Autodesk Inventor part; units mm, degrees
ref_plane "YZ Plane" through (0, 0, 0) normal (1, 0, 0) x (0, 1, 0)
ref_plane "XZ Plane" through (0, 0, 0) normal (0, 1, 0) x (-1, 0, 0)
ref_plane "XY Plane" through (0, 0, 0) normal (0, 0, 1) x (1, 0, 0)
sketch "Эскиз1" plane through (0, 0, 0) normal (0, 1, 0) x (-1, 0, 0)
  line L0 (30, 60) -> (-30, 60)
  line L1 (-30, 60) -> (-30, -60)
  line L2 (-30, -60) -> (30, -60)
  line L3 (30, -60) -> (30, 60)
  point P0 (0, 0)
  dimension "d0" = 60
  dimension "d1" = 120
extrude "Выдавливание1" add sketch "Эскиз1" along normal blind 80
sketch "Эскиз2" plane through (0, 0, 0) normal (1, 0, 0) x (0, 1, 0)
  line L0 (80, 60) -> (80, -60)
  line L1 (80, -30) -> (70, -30)
  line L2 (80, -30) -> (90, -30) construction
  line L3 (70, -30) -> (70, -10)
  line L4 (70, -10) -> (60, -10)
  line L5 (60, -10) -> (60, 10)
  line L6 (60, 10) -> (70, 10)
  line L7 (70, 10) -> (70, 30)
  line L8 (70, 30) -> (80, 30)
extrude "Выдавливание2" cut sketch "Эскиз2" against normal mid plane 80
sketch "Эскиз3" plane through (0, 0, 0) normal (1, 0, 0) x (0, 1, 0)
  line L0 (0, 60) -> (0, -60)
  line L1 (0, -15) -> (10, -15)
  line L2 (0, -15) -> (10, -15) construction
  line L3 (10, -15) -> (10, -25)
  line L4 (10, -25) -> (15, -25)
  line L5 (0, -15) -> (0, 15)
  line L6 (0, 15) -> (10, 15)
  line L7 (10, 15) -> (10, 25)
  line L8 (10, 25) -> (15, 25)
  arc A0 (15, -25) -> (15, 25) centre (15, 0) ccw
  point P0 (0, 0)
  dimension "d20" = 10
  dimension "d21" = 0
  dimension "d22" = 30
extrude "Выдавливание3" cut sketch "Эскиз3" against normal mid plane 80
sketch "Эскиз4" plane through (0, 0, 0) normal (0, 1, 0) x (-1, 0, 0)
  circle A0 centre (0, 0) radius 25
  dimension "d25" = 50
extrude "Выдавливание4" cut sketch "Эскиз4" along normal blind 80
sketch "Эскиз5" plane through (30, 0, -60) normal (1, 0, 0) x (0, 0, -1)
  line L0 (-120, 0) -> (-120, 80)
  line L1 (-120, 20) -> (-100, 20)
  line L2 (-120, 20) -> (-100, 20) construction
  line L3 (-100, 20) -> (-100, 80)
  line L4 (-120, 80) -> (-90, 80)
  line L5 (0, 0) -> (0, 80)
  line L6 (0, 20) -> (-20, 20)
  line L7 (0, 20) -> (20, 20) construction
  line L8 (-20, 20) -> (-20, 80)
  line L9 (0, 80) -> (-30, 80)
  point P0 (-60, 0)
  dimension "d28" = 20
  dimension "d29" = 0
  dimension "d30" = 20
  dimension "d31" = 180
extrude "Выдавливание5" cut sketch "Эскиз5" against normal blind 25
sketch "Эскиз6" plane through (-30, 0, 60) normal (-1, 0, 0) x (0, 0, 1)
  line L0 (-120, 0) -> (-120, 80)
  line L1 (-120, 20) -> (-100, 20)
  line L2 (-120, 20) -> (-100, 20)
  line L3 (-100, 20) -> (-100, 80)
  line L4 (-120, 80) -> (-90, 80)
  line L5 (-20, 20) -> (0, 20)
  line L6 (0, 20) -> (-20, 20)
  line L7 (-20, 80) -> (-20, 20)
  line L8 (-20, 20) -> (-20, 80)
  line L9 (-20, 80) -> (-30, 80)
  line L10 (-30, 80) -> (0, 80)
  line L11 (-20, 80) -> (0, 80)
  line L12 (0, 20) -> (0, 80)
  line L13 (0, 80) -> (0, 20)
  point P0 (-60, 0)
extrude "Выдавливание6" cut sketch "Эскиз6" against normal blind 25
sketch "Эскиз7" plane through (5, 0, -60) normal (1, 0, 0) x (0, 0, -1)
  line L0 (-20, 80) -> (-20, 20)
  line L1 (-20, 20) -> (0, 20)
  line L2 (-20, 80) -> (0, 20)
  line L3 (0, 20) -> (-20, 20)
  line L4 (0, 80) -> (-20, 80)
  line L5 (-20, 20) -> (-20, 80)
  line L6 (0, 20) -> (0, 80)
  line L7 (0, 80) -> (0, 20)
  point P0 (-60, 0)
extrude "Выдавливание7" cut sketch "Эскиз7" against normal blind 25 contours L4 L6 L2
sketch "Эскиз8" plane through (5, 0, -60) normal (1, 0, 0) x (0, 0, -1)
  line L0 (-120, 20) -> (-120, 80)
  line L1 (-100, 80) -> (-120, 20)
  line L2 (-120, 20) -> (-120, 80)
  line L3 (-120, 80) -> (-100, 80)
  line L4 (-120, 80) -> (-100, 80)
  point P0 (-60, 0)
extrude "Выдавливание8" cut sketch "Эскиз8" against normal blind 25
Verification items for the finished model (mm, model axes). A direction names the side the tool comes from. Round coordinates to 2 decimals unless told otherwise and drop trailing zeros. Loops run counter-clockwise (first coordinate to the right, second up) from the corner with the lowest first, then second, coordinate; pieces in that order, holes last. Notation, with made-up numbers: (56, 23.5) - (69, 23.5) arc R24 ccw to (69, 37.5) - close; hole circle Ø8 at (-38.5, 63.5). An arc over 180 degrees is marked (long way). Answer in a Markdown table with one row per item. Add a question column.
Q1. Section check C-C on x = -10. Enter the section's corners in (y, z), plus the area to 3 significant figures.
Q2. Tool access check on faces 5 (the face through (5, 37, 46)), 6 (the face through (27, 65, -10)), 7 (the face through (0, 12, 25)), 8 (the face through (5, 37, -45)), 9 (the face through (-18, 50, 40)). Record the directions out of +Z, -Z, +X, -X, +Y, -Y that give a thin tool (end or side, any length) a straight path to the whole face; none if there is none.
Q3. Section check A-A on y = 6. Enter the section's corners in (x, z).
Q4. Section check B-B on z = 0. Enter the section's corners in (x, y).
Q5. Gauge pin test, flat ends, axial feed: pin 1 (8 mm diameter, centred on x = 26.5, z = -1.5, fed in from +Y); pin 2 (4 mm diameter, centred on x = 5, y = 31.5, fed in from -Z); pin 3 (3 mm diameter, centred on x = -19, y = 33.5, fed in from +Z). Record the tip position at first contact, or that the pin passes through.
Q6. Section check D-D on z = 50. Enter the section's corners in (x, y), plus the area to 3 significant figures.
Q7. Material ranges on line 1 (X direction, y = 56, z = 0); line 2 (Y direction, x = -10, z = -45.5); line 3 (Z direction, x = 0, y = 44), recorded low to high.
Q8. Release check for a two-part mould opening along Y. For faces 1 (the face through (-21, 10, -21)), 2 (the face through (-18, 50, -40)), 3 (the face through (22, 10, -21)), 4 (the face through (18, 20, 50)) record: pulls with the +Y half, pulls with the -Y half, needs draft (parallel to the pull), parting line crosses it, or undercut.
Found:
| question | item | result |
|---|---|---|
| 1 | outline | (0, -60) - (20, -60) - (20, -40) - (80, -40) - (80, -30) - (70, -30) - (70, -22.91) - (25, -22.91) arc R25 cw to (15, -25) - (10, -25) - (10, -22.91) - (0, -22.91) - close; (0, 22.91) - (10, 22.91) - (10, 25) - (15, 25) arc R25 cw to (25, 22.91) - (70, 22.91) - (70, 30) - (80, 30) - (80, 40) - (20, 40) - (20, 60) - (0, 60) - close |
| 1 | area | 3,340 mm² |
| 2 | face 5 | +Z, +X, +Y |
| 2 | face 6 | +X, -X, +Y |
| 2 | face 7 | +X, -X |
| 2 | face 8 | -Z, +X, +Y |
| 2 | face 9 | +Z, -X, +Y |
| 3 | outline | (-30, -60) - (30, -60) - (30, -15) - (20, -15) arc R25 cw to (-20, -15) - (-30, -15) - close; (-30, 15) - (-20, 15) arc R25 cw to (20, 15) - (30, 15) - (30, 60) - (-30, 60) - close |
| 4 | outline | (-30, 40) - (-25, 40) - (-25, 60) - (-30, 60) - close; (25, 40) - (30, 40) - (30, 60) - (25, 60) - close |
| 5 | pin 1 | stops at y = 60 |
| 5 | pin 2 | stops at z = -56.83 |
| 5 | pin 3 | stops at z = 40 |
| 6 | outline | (-30, 0) - (30, 0) - (30, 20) - (5, 20) - (5, 50) - (-5, 50) - (-5, 20) - (-30, 20) - close |
| 6 | area | 1,500 mm² |
| 7 | line 1 | x = -30 to -25, 25 to 30 |
| 7 | line 2 | y = 0 to 20 |
| 7 | line 3 | z = -52 to -25, 25 to 52 |
| 8 | face 1 | undercut |
| 8 | face 2 | needs draft |
| 8 | face 3 | undercut |
| 8 | face 4 | pulls with the +Y half |
